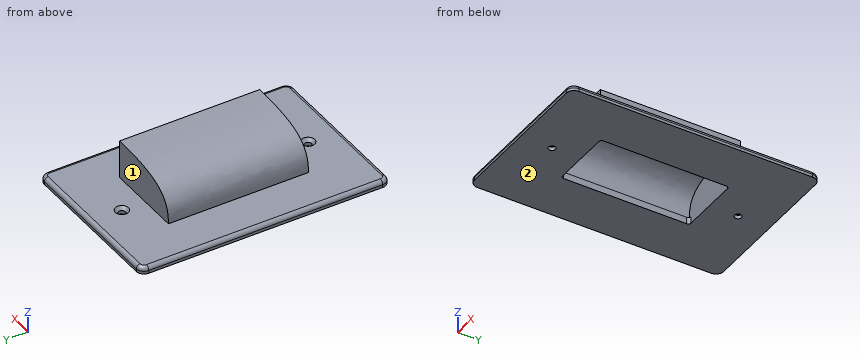
```python
from build123d import *

# Parameters (mm, degrees)
SKETCH_W        = 84.8
SKETCH_H        = 129.6
SKETCH_R        = 1.8
SKETCH_W_2      = 33.2
SKETCH_H_2      = 66.8
PAD_DEPTH       = 3.5
CHAMFER_SIZE    = 1.6
FILLET_R        = 4
FILLET001_R     = 2
FILLET002_R     = 1.4
PAD001_DEPTH    = 20
POCKET_START    = -3
POCKET_DEPTH    = 66.8
POCKET001_DEPTH = 101.201


with BuildPart() as part:
    # Sketch → Pad (new body)
    with BuildSketch(Plane.XY):
        Rectangle(SKETCH_W, SKETCH_H)
        with Locations((0, 48.4)):
            Circle(SKETCH_R, mode=Mode.SUBTRACT)
        with Locations((0, -48.4)):
            Circle(SKETCH_R, mode=Mode.SUBTRACT)
        Rectangle(SKETCH_W_2, SKETCH_H_2, mode=Mode.SUBTRACT)
    extrude(amount=PAD_DEPTH)

    # Chamfer
    chamfer_edges = [part.edges().sort_by_distance(p)[0] for p in [
        (-1.8, -48.4, 3.5),
        (-1.8, 48.4, 3.5),
    ]]
    chamfer(chamfer_edges, length=CHAMFER_SIZE)

    # Fillet
    fillet_edges = [part.edges().sort_by_distance(p)[0] for p in [
        (42.4, 64.8, 1.75),
        (-42.4, 64.8, 1.75),
        (42.4, -64.8, 1.75),
        (-42.4, -64.8, 1.75),
    ]]
    fillet(fillet_edges, radius=FILLET_R)

    # Fillet001
    fillet001_edges = [part.edges().sort_by_distance(p)[0] for p in [
        (-41.228427, -63.628427, 3.5),
        (0, -64.8, 3.5),
        (41.228427, -63.628427, 3.5),
        (42.4, 0, 3.5),
        (41.228427, 63.628427, 3.5),
        (0, 64.8, 3.5),
        (-41.228427, 63.628427, 3.5),
        (-42.4, 0, 3.5),
    ]]
    fillet(fillet001_edges, radius=FILLET001_R)

    # Fillet002
    fillet002_edges = [part.edges().sort_by_distance(p)[0] for p in [
        (-16.6, -33.4, 1.75),
        (16.6, 33.4, 1.75),
        (16.6, -33.4, 1.75),
        (-16.6, 33.4, 1.75),
    ]]
    fillet(fillet002_edges, radius=FILLET002_R)

    # Sketch001 (on Face20 of Fillet002) → Pad001 (join)
    with BuildSketch(Plane.XY.offset(3.5)):
        Polygon((21.2, 36.4), (-19.6, 36.4), (-19.6, -36.4), (21.2, -36.4), (21.2, -33.4), (21.2, 33.4), align=None)
    extrude(amount=PAD001_DEPTH)

    # Sketch002 (on Face35 of Pad001) → Pocket (cut)
    with BuildSketch(Plane.XZ.offset(36.4).offset(POCKET_START)):
        with BuildLine():
            Line((21.2, 20.5), (21.2, 3.5))
            Line((21.2, 3.5), (-16.6, 3.5))
            add(Edge.make_bspline(
                [(-16.6, 3.5), (-16.6, 13.299617), (-13.358306, 20.5), (21.2, 20.5)],
                knots=[0, 0, 0, 0, 1, 1, 1, 1], degree=3))
        make_face()
    extrude(amount=-POCKET_DEPTH, mode=Mode.SUBTRACT)

    # Sketch003 (on Face43 of Pocket) → Pocket001 (cut, through all)
    with BuildSketch(Plane.XZ.offset(36.4)):
        with BuildLine():
            add(Edge.make_bspline(
                [(-19.6, 3.5), (-19.6, 17.472133), (-10.864879, 23.5), (21.2, 23.5)],
                knots=[0, 0, 0, 0, 1, 1, 1, 1], degree=3))
            Line((21.2, 23.5), (-19.6, 23.5))
            Line((-19.6, 23.5), (-19.6, 3.5))
        make_face()
    extrude(amount=-POCKET001_DEPTH, mode=Mode.SUBTRACT)


solid = part.part
```
Build history of the part. All positions in model axes, mm. Face numbers are marked on the shaded views. A direction names the side the tool comes from. Round coordinates to 2 decimals unless told otherwise and drop trailing zeros. Order: outer loops, then holes, each group sorted by start corner. A loop starts at its lowest first (then second) coordinate and runs counter-clockwise, first axis right, second up. Notation, with made-up numbers: (81, -1.5) - (95, -1.5) arc R26 cw to (95, 36.5) - close; hole circle Ø5 at (60, 44). An arc over 180 degrees is marked (long way). Use a Markdown table: item, result.
1) Flat gauge pins, fed straight in: pin 1 Ø8 at (x, y) = (-8, 6) entering from -Z; pin 2 Ø3 at (y, z) = (-33, 17) entering from -X; pin 3 Ø3 at (x, y) = (-16.5, 10.5) entering from +Z; pin 4 Ø3 at (x, y) = (0, 48.4) entering from +Z. Where does each tip first touch, or does it go through?
Recorded:
| item | result |
|---|---|
| pin 1 | stops at z = 14.79 |
| pin 2 | stops at x = -15.61 |
| pin 3 | stops at z = 16.11 |
| pin 4 | passes through |
2) Saw through at B-B on x = -28.5. Write the cut outline in (y, z), and give its area (3 significant figures).
Recorded:
| item | result |
|---|---|
| outline | (-64.8, 0) - (64.8, 0) - (64.8, 1.5) arc R2 ccw to (62.8, 3.5) - (-62.8, 3.5) arc R2 ccw to (-64.8, 1.5) - close |
| area | 452 mm² |
3) Saw through at C-C on x = 0. Give the number of separate pieces and of enclosed holes in the cut face, and give its area (3 significant figures).
Recorded:
| item | result |
|---|---|
| separate pieces | 3 |
| enclosed holes | 0 |
| area | 502 mm² |
4) Tool access for the marked faces 1 and 2: list every direction of +Z, -Z, +X, -X, +Y, -Y with a clear straight run to the whole face (end or side of a thin tool).
Recorded:
| item | result |
|---|---|
| face 1 | +Z, +X, -X, +Y |
| face 2 | -Z, +X, -X, +Y, -Y |
5) Wall check: L1, parallel to Y at x = 0, z = 0.7; L2, parallel to Y at x = 13.5, z = 7; L3, parallel to Z at x = 19, y = 23.5. Give the ranges that are in metal, low to high.
Recorded:
| item | result |
|---|---|
| L1 | y = -64.8 to -50.2, -46.6 to -33.4, 33.4 to 46.6, 50.2 to 64.8 |
| L2 | y = -36.4 to -33.4, 33.4 to 36.4 |
| L3 | z = 0 to 3.5, 20.49 to 23.49 |
6) Saw through at A-A on y = -48.4. Write the cut outline in (x, z), and give its area (3 significant figures).
Recorded:
| item | result |
|---|---|
| outline | (-42.4, 0) - (-1.8, 0) - (-1.8, 1.9) - (-3.4, 3.5) - (-40.4, 3.5) arc R2 ccw to (-42.4, 1.5) - close; (1.8, 0) - (42.4, 0) - (42.4, 1.5) arc R2 ccw to (40.4, 3.5) - (3.4, 3.5) - (1.8, 1.9) - close |
| area | 280 mm² |
